from build123d import *

# Parameters (mm, degrees)
BOSS_EXTRUDE1_DEPTH = 80
SKETCH2_W           = 4.8
SKETCH2_H           = 4.8
BOSS_EXTRUDE2_DEPTH = 150
SKETCH3_W           = 11
SKETCH3_H           = 20
CUT_EXTRUDE1_DEPTH  = 200.226102707
FILLET1_R           = 5


with BuildPart() as part:
    # Sketch1 → Boss-Extrude1 (new body)
    with BuildSketch(Plane.XY):
        Polygon((-80, 0), (70, 0), (70, 100), (60, 100), (60, 10), (-80, 10), align=None)
    extrude(amount=BOSS_EXTRUDE1_DEPTH)

    # Sketch2 → Boss-Extrude2 (add)
    with BuildSketch(Plane(origin=(70, 0, 0), x_dir=(0, 0, -1), z_dir=(1, 0, 0))):
        with Locations((-82.4, 7.4)):
            Rectangle(SKETCH2_W, SKETCH2_H)
        with Locations((2.4, 7.4)):
            Rectangle(SKETCH2_W, SKETCH2_H)
    extrude(amount=-BOSS_EXTRUDE2_DEPTH)

    # Sketch3 → Cut-Extrude1 (cut, through all)
    with BuildSketch(Plane(origin=(70, 0, 0), x_dir=(0, 0, -1), z_dir=(1, 0, 0))):
        Polygon((-40, 100), (-50, 100), (-50, 95), (-30, 95), (-30, 100), align=None)
        with Locations((-74.5, 90)):
            Rectangle(SKETCH3_W, SKETCH3_H)
        with Locations((-5.5, 90)):
            Rectangle(SKETCH3_W, SKETCH3_H)
    extrude(amount=-CUT_EXTRUDE1_DEPTH, mode=Mode.SUBTRACT)

    # Fillet1
    fillet1_edges = [part.edges().sort_by_distance(p)[0] for p in [
        (70, 0, 40),
    ]]
    fillet(fillet1_edges, radius=FILLET1_R)


solid = part.part
Model file for the job. Use its own axes, mm. A direction names the side the tool comes from. Round coordinates to 2 decimals unless told otherwise and drop trailing zeros. Order: outer loops, then holes, each group sorted by start corner. A loop starts at its lowest first (then second) coordinate and runs counter-clockwise, first axis right, second up.
(1) Band-saw the part on D-D (z = 6). List the corners of the cut face in (x, y), then the cut area to 3 significant figures.
(2) Pull direction Z, two halves, no side cores. Call faces 4 (the face through (-4, 7, 84.8)), 5 (the face through (65, 80, 75)), 6 (the face through (65, 97, 30)): released by +Z, released by -Z, zero draft, split by the parting line, or undercut.
(3) 3-axis set-ups, long thin cutter, end or side, ignore diameter. For faces 1 (the face through (-4, 5, 82)), 2 (the face through (65, 98, 50)), 3 (the face through (61, 45, 0)): which of +Z, -Z, +X, -X, +Y, -Y reach the whole face in a straight line?
(4) Pin check, flat tips, straight feed: pin 1 (5 mm diameter, centred on x = 66.5, z = 5.5, fed in from +Y); pin 2 (6 mm diameter, centred on x = -46, z = 25, fed in from +Y); pin 3 (1.5 mm diameter, centred on x = 66.5, y = 98, fed in from -Z). Stop position of each tip, or through.
(5) Band-saw the part on B-B (z = 45.5). List the corners of the cut face in (x, y).
(6) Band-saw the part on C-C (y = 43). List the corners of the cut face in (x, z), then the cut area to 3 significant figures.
(7) Band-saw the part on A-A (x = -7). List the corners of the cut face in (y, z), then the cut area to 3 significant figures.
(8) Drill centre lines: line 1 (Z direction, x = 64.5, y = 43); line 2 (X direction, y = 12, z = 43.5); line 3 (Y direction, x = 49, z = -1). Where is each one in solid material? Low to high.
Verdict:
1. outline: (-80, 0) - (65, 0) arc R5 ccw to (70, 5) - (70, 80) - (60, 80) - (60, 10) - (-80, 10) - close
1. area: 2,190 mm2
2. face 4: released by +Z
2. face 5: zero draft
2. face 6: undercut
3. face 1: +Z, +X, -X, -Y
3. face 2: +X, -X, +Y
3. face 3: -Z, +X, -X, +Y
4. pin 1: stops at y = 80
4. pin 2: stops at y = 10
4. pin 3: stops at z = 11
5. outline: (-80, 0) - (65, 0) arc R5 ccw to (70, 5) - (70, 95) - (60, 95) - (60, 10) - (-80, 10) - close
6. outline: (60, 0) - (70, 0) - (70, 80) - (60, 80) - close
6. area: 800 mm2
7. outline: (0, 0) - (5, 0) - (5, -4.8) - (9.8, -4.8) - (9.8, 0) - (10, 0) - (10, 80) - (9.8, 80) - (9.8, 84.8) - (5, 84.8) - (5, 80) - (0, 80) - close
7. area: 846 mm2
8. line 1: z = 0 to 80
8. line 2: x = 60 to 70
8. line 3: y = 5 to 9.8
